The listing builds one solid part. Answer for the finished solid, in the listing's coordinates (mm). Coordinates: 2 decimals unless noted, no trailing zeros. Write each loop counter-clockwise with the first axis right and the second up, starting at its lowest first coordinate (ties: lowest second). Pieces come first, ordered by that corner, then holes. Notation, with made-up numbers: M -17,-8.75 L 26,-8.75 A26 cw 26,9.25 Z; hole C -19,47.5 d11. An arc over 180 degrees is marked long. Answer as a JSON object with one key per item and string values. Group by question number.
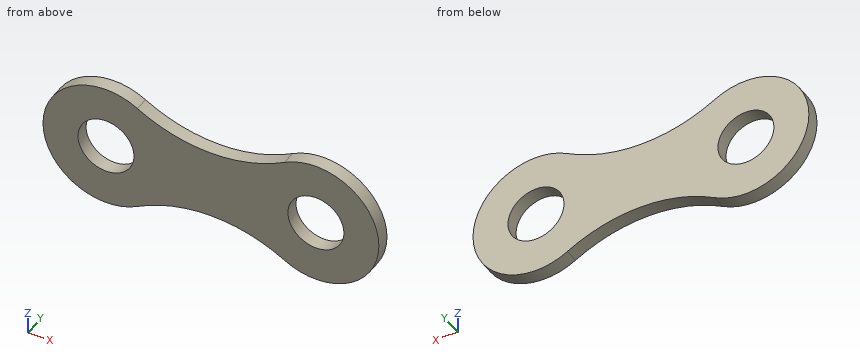
from build123d import *

# Parameters (mm, degrees)
SKIZZE2_R          = 2
BASIS_BLECH1_DEPTH = 1


# Sheet-metal steps are written as plain solids
with BuildPart() as part:
    # Skizze2 → Basis-Blech1 (new body)
    with BuildSketch(Plane(origin=(0, 0, 0), x_dir=(1, 0, 0), z_dir=(0, 1, 0))):
        with BuildLine():
            ThreePointArc((-5.254458339, 3.899684942), (0, 2.494976886), (5.254458339, 3.899684942))
            ThreePointArc((5.254458339, 3.899684942), (12, 0), (5.254458339, -3.899684942))
            ThreePointArc((5.254458339, -3.899684942), (0, -2.494976886), (-5.254458339, -3.899684942))
            ThreePointArc((-5.254458339, -3.899684942), (-12, 0), (-5.254458339, 3.899684942))
        make_face()
        with Locations(Location((-7.5, 0, 0), (0, 0, 270))):
            Circle(SKIZZE2_R, mode=Mode.SUBTRACT)
        with Locations(Location((7.5, 0, 0), (0, 0, 270))):
            Circle(SKIZZE2_R, mode=Mode.SUBTRACT)
    extrude(amount=-BASIS_BLECH1_DEPTH)


solid = part.part
Item 1: A cutting plane is placed at C-C, the plane y = -0.5. Write down the section's boundary in (x, z), and give its area (3 significant figures).
Item 2: A cutting plane is placed at B-B, the plane z = 3.5. Write down the section's boundary in (x, y), and give its area (3 significant figures).
Item 3: A cutting plane is placed at D-D, the plane z = 0.5. Write down the section's boundary in (x, y).
Item 4: A flat-ended cylindrical pin translates along its axis: pin 1 Ø3 at (x, z) = (-7.5, 0) entering from +Y. Find the tip coordinate at first contact, or state that the pin passes through.
Item 5: A cutting plane is placed at A-A, the plane x = 7.5. Write down the section's boundary in (y, z).
Item 6: Consider L1, parallel to X at y = -0.6, z = 1.5; L2, parallel to Z at x = 0, y = -0.9; L3, parallel to X at y = -0.7, z = -3.25. Determine where each line is inside the solid, lowest interval first. Write a range as from..to.
Answer:
{
 "1": {"outline": "M -5.25,-3.9 A10.53 cw 5.25,-3.9 A4.5 ccw long 5.25,3.9 A10.53 cw -5.25,3.9 A4.5 ccw long Z; hole C -7.5,0 d4; hole C 7.5,0 d4", "area": "139 mm2"},
 "2": {"outline": "M -10.33,-1 L -4.49,-1 L -4.49,0 L -10.33,0 Z; M 4.49,-1 L 10.33,-1 L 10.33,0 L 4.49,0 Z", "area": "11.7 mm2"},
 "3": {"outline": "M -11.97,-1 L -9.44,-1 L -9.44,0 L -11.97,0 Z; M -5.56,-1 L 5.56,-1 L 5.56,0 L -5.56,0 Z; M 9.44,-1 L 11.97,-1 L 11.97,0 L 9.44,0 Z"},
 "4": {"pin 1": "through"},
 "5": {"outline": "M -1,-4.5 L 0,-4.5 L 0,-2 L -1,-2 Z; M -1,2 L 0,2 L 0,4.5 L -1,4.5 Z"},
 "6": {"L1": "-11.74..-8.82, -6.18..6.18, 8.82..11.74", "L2": "-2.49..2.49", "L3": "-10.61..-3.92, 3.92..10.61"}
}
